Input: part model. Units: mm. Frame: model coordinates. Face numbers are marked on the shaded views. A direction names the side the tool comes from. Give positions to 0.01 mm unless a question says otherwise; leave off trailing zeros. Write each loop counter-clockwise with the first axis right and the second up, starting at its lowest first coordinate (ties: lowest second). Pieces come first, ordered by that corner, then holes. Notation, with made-up numbers: (49.5, 0) -> (75.5, 0) arc R15 ccw to (75.5, 14) -> close; hole circle Ø10 at (-27, -8). An arc over 180 degrees is marked (long way). Return JSON: item names as keys, results as strings. Group by question number.
Item 1: Pin query (flat end, axial travel): P1, Ø0.7, axis at y = -3, z = 3, coming from the +X side; P2, Ø1, axis at x = -1, z = 5, coming from the -Y side; P3, Ø1.9, axis at y = -3, z = 2.5, coming from the -X side. Return the tip coordinate at first contact, or that it passes through.
Item 2: Set-up query: the marked faces 4 and 5. Return all of +Z, -Z, +X, -X, +Y, -Y with unobstructed straight access to the full face (end or side cutting, diameter ignored); none if empty.
Item 3: Line query: line 1 (Z direction, x = 0, y = -0.85); line 2 (X direction, y = -2.9, z = 5); line 3 (X direction, y = -3, z = 1). Output: solid intervals per line, ascending. Write a range as [from, to].
Item 4: Section A-A, the plane x = 0. Return loops of the section in (y, z).
Item 5: Section C-C, the plane y = -0.5. Return loops of the section in (x, z), then the cut area to 3 significant figures.
Item 6: Mould query, pull axis X, two halves, no side actions, for the marked faces 1, 2 and 3. Classes: released by +X, released by -X, zero draft, split by the parting line, or undercut.
Item 7: Section B-B, the plane z = 2.25. Return loops of the section in (x, y).
Item 8: Section D-D, the plane y = -2.85. Return loops of the section in (x, z), then the cut area to 3 significant figures.
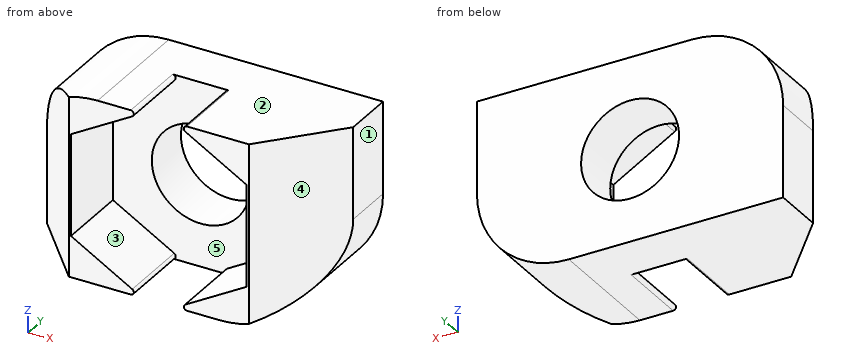
from build123d import *

# Parameters (mm, degrees)
PAD_DEPTH       = 6
SKETCH001_R     = 1.6
POCKET_DEPTH    = 4.001
POCKET001_DEPTH = 2.36
FILLET_R        = 0.1
FILLET001_R     = 3


with BuildPart() as part:
    # Sketch → Pad (new body)
    with BuildSketch(Plane.XY):
        Polygon((0, 0), (-5, 0), (-5, -1.68), (-2.94, -4), (0, -4), (2.94, -4), (5, -1.68), (5, 0), align=None)
    extrude(amount=PAD_DEPTH)

    # Sketch001 (on Face5 of Pad) → Pocket (cut, through all)
    with BuildSketch(Plane.XZ.offset(4)):
        with Locations((0, 3)):
            Circle(SKETCH001_R)
    extrude(amount=-POCKET_DEPTH, mode=Mode.SUBTRACT)

    # Sketch002 (on Face8 of Pocket) → Pocket001 (cut)
    with BuildSketch(Plane.XZ.offset(4)):
        Polygon((-2.87, 4.656995), (-2.87, 1.343005), (0, -0.313991), (2.87, 1.343005), (2.87, 4.656995), (0, 6.313991), align=None)
    extrude(amount=-POCKET001_DEPTH, mode=Mode.SUBTRACT)

    # Fillet
    fillet_edges = [part.edges().sort_by_distance(p)[0] for p in [
        (-0.543848, -2.82, 6),
        (0.543848, -2.82, 6),
        (0.543848, -2.82, 0),
        (-0.543848, -2.82, 0),
    ]]
    fillet(fillet_edges, radius=FILLET_R)

    # Fillet001
    fillet001_edges = [part.edges().sort_by_distance(p)[0] for p in [
        (5, -0.84, 0),
        (-5, -0.84, 6),
    ]]
    fillet(fillet001_edges, radius=FILLET001_R)


solid = part.part
Answer below:
{
 "1": {"P1": "stops at x = 4.14", "P2": "stops at y = -1.64", "P3": "stops at x = -4.67"},
 "2": {"face 4": "+Z, -Z, +X, -Y", "face 5": "-Y"},
 "3": {"line 1": "z = [0, 1.4], [4.6, 6]", "line 2": "x = [-3.92, -2.28], [2.28, 3.92]", "line 3": "x = [-3.83, -2.28], [2.28, 3.83]"},
 "4": {"outline": "(-1.64, 0) -> (0, 0) -> (0, 1.4) -> (-1.64, 1.4) -> close; (-1.64, 4.6) -> (0, 4.6) -> (0, 6) -> (-1.64, 6) -> close"},
 "5": {"outline": "(-5, 0) -> (2, 0) arc R3 ccw to (5, 3) -> (5, 6) -> (-2, 6) arc R3 ccw to (-5, 3) -> close; hole circle Ø3.2 at (0, 3)", "area": "48.1 mm2"},
 "6": {"face 1": "released by +X", "face 2": "zero draft", "face 3": "undercut"},
 "7": {"outline": "(-5, -1.68) -> (-2.94, -4) -> (-2.87, -4) -> (-2.87, -1.64) -> (-1.41, -1.64) -> (-1.41, 0) -> (-5, 0) -> close; (1.41, -1.64) -> (2.87, -1.64) -> (2.87, -4) -> (2.94, -4) -> (4.9, -1.79) -> (4.9, 0) -> (1.41, 0) -> close"},
 "8": {"outline": "(-3.96, 0) -> (-0.92, 0) arc R0.1 ccw to (-0.87, 0.19) -> (-2.87, 1.34) -> (-2.87, 4.66) -> (-0.87, 5.81) arc R0.1 ccw to (-0.92, 6) -> (-2, 6) arc R3 ccw to (-3.96, 5.27) -> close; (0.87, 0.19) arc R0.1 ccw to (0.92, 0) -> (2, 0) arc R3 ccw to (3.96, 0.73) -> (3.96, 6) -> (0.92, 6) arc R0.1 ccw to (0.87, 5.81) -> (2.87, 4.66) -> (2.87, 1.34) -> close", "area": "18.3 mm2"}
}
